Autodesk Inventor part; units mm, degrees
ref_plane "Work Plane1" through (-2.5, 0, -1.5) normal (0, 0, -1) x (-1, 0, 0)
ref_plane "Work Plane2" through (3.625, 2, -19.5) normal (0, 0, -1) x (-1, 0, 0)
ref_plane "YZ Plane" through (0, 0, 0) normal (1, 0, 0) x (0, 1, 0)
sketch "Sketch2" plane through (0, 0, 0) normal (0, 0, 1) x (1, 0, 0)
  circle A0 centre (2.5, 0) radius 1.5
  circle A1 centre (-2.5, 0) radius 1.5
  arc A2 (-1.9231, 1.3846) -> (1.9231, 1.3846) centre (0, 6) ccw
  arc A3 (1.9231, -1.3846) -> (-1.9231, -1.3846) centre (0, -6) ccw
  circle A4 centre (2.5, 0) radius 0.75
  circle A5 centre (-2.5, 0) radius 0.75
  point P0 (0, 0)
  dimension "d0" = 3
  dimension "d1" = 3
  dimension "d2" = 6
  dimension "d3" = 6
  dimension "d4" = 2.5
  dimension "d5" = 2.5
  dimension "d6" = 1.5
  dimension "d7" = 1.5
extrude "Extrusion2" add sketch "Sketch2" along normal blind 0.8
sketch "Sketch3" plane through (0, 0, 0) normal (0, 0, -1) x (-1, 0, 0)
  arc A0 (1.9231, -1.3846) -> (-1.9231, -1.3846) centre (0, -6) ccw
  arc A1 (1.9231, -1.3846) -> (1.9231, 1.3846) centre (2.5, 0) ccw
  arc A2 (-1.9231, 1.3846) -> (1.9231, 1.3846) centre (0, 6) ccw
  arc A3 (-1.9231, 1.3846) -> (-1.9231, -1.3846) centre (-2.5, 0) ccw
  circle A4 centre (-2.5, 0) radius 0.75
  circle A5 centre (2.5, 0) radius 0.75
  circle A6 centre (-2.5, 0) radius 1.125
  line L0 (-3.625, 2) -> (-1.375, 2)
  line L1 (-1.375, 2) -> (-1.375, 0)
  line L2 (-3.625, 0) -> (-3.625, 2)
  line L3 (0, -8.4) -> (0, 8.4)
  point P0 (0, 0)
  point P1 (-3.4922, 1.125)
  point P2 (-3.625, 0.9922)
  point P3 (-1.375, 1.1928)
  dimension "d12" = 2.25
  dimension "d16" = 1.5
  dimension "d20" = 2
extrude "Extrusion3" add sketch "Sketch3" along normal blind 1.5 contours L2 L0 L1 A2 A3 | A3 A2 L1 A6 L2 | A6
mirror "Mirror1" about plane through (0, 0, 0) normal (1, 0, 0) of "Extrusion3"
ref_plane "Work Plane1" through (-2.5, 0, -1.5) normal (0, 0, -1) x (-1, 0, 0)
mirror "Mirror2" about plane through (-2.5, 0, -1.5) normal (0, 0, -1) of "Extrusion3", "Mirror1", "Extrusion2"
sketch "Sketch4" plane through (1.375, 2, 0) normal (0, 1, 0) x (1, 0, 0)
  line L0 (-5, -4.5) -> (2.25, -4.5)
  line L1 (2.25, -4.5) -> (2.25, 1.5)
  line L2 (-5, 1.5) -> (-5, -4.5)
  line L3 (-2.75, 0) -> (-5, 0)
  line L4 (-2.75, 0) -> (-2.75, 3)
  line L5 (-2.75, 3) -> (-5, 3)
  line L6 (-5, 0) -> (-5, 3)
  line L7 (0, 0) -> (2.25, 0)
  line L8 (2.25, 0) -> (2.25, 3)
  line L9 (0, 3) -> (2.25, 3)
  line L10 (0, 0) -> (0, 3)
  line L11 (-5, 0) -> (-5, 3)
  line L12 (2.25, 0) -> (2.25, 3)
  line L13 (2.25, 1.5) -> (-5, 1.5)
  line L14 (2.25, 1.5) -> (-5, 1.5)
  line L15 (-5, 1.5) -> (-5, 19.5)
  line L16 (-5, 19.5) -> (2.25, 19.5)
  line L17 (2.25, 19.5) -> (2.25, 1.5)
  point P0 (-1.375, 0)
  point P1 (2.25, 1.5)
  point P2 (2.25, 3)
  dimension "d22" = 18
  dimension "d23" = 6
extrude "Extrusion4" add sketch "Sketch4" along normal blind 1.5
sketch "Sketch5" plane through (1.375, 3.5, 0) normal (0, 1, 0) x (1, 0, 0)
  line L0 (1.5, -1.5) -> (-4.25, -1.5)
  line L1 (-4.25, -1.5) -> (-4.25, -3.5)
  line L2 (-4.25, -3.5) -> (1.5, -3.5)
  line L3 (1.5, -3.5) -> (1.5, -1.5)
  line L4 (-5, -4.5) -> (2.25, -4.5)
  line L5 (2.25, -4.5) -> (2.25, 19.5)
  line L6 (2.25, 19.5) -> (-5, 19.5)
  line L7 (-5, 19.5) -> (-5, -4.5)
  point P0 (-1.375, 0)
  dimension "d26" = 5.75
  dimension "d27" = 7.25
  dimension "d28" = 2
  dimension "d29" = 0.75
  dimension "d30" = 1
extrude "Extrusion5" add sketch "Sketch5" along normal blind 1 contours L3 L2 L1 L0
pattern_linear "Rectangular Pattern1" count 5 spacing 4 along (0, 0, -1) of "Extrusion5"
ref_plane "Work Plane2" through (3.625, 2, -19.5) normal (0, 0, -1) x (-1, 0, 0)
mirror "Mirror3" about plane through (3.625, 2, -19.5) normal (0, 0, -1) of "Extrusion4", "Extrusion3", "Mirror1", "Extrusion2", "Mirror2", "Extrusion5", "Rectangular Pattern1"
equation "\"d1\" = d0"
equation "\"d7\" = d6"
equation "\"d12\" = d16 + 0.5 * d13"
equation "\"d29\" = -0.5 * d26 + 0.5 * d27"
properties part number "McCrea_CHAIN_INK_WALLE"
Here's how the part is built. I have some questions about the finished solid (model axes, mm). A direction names the side the tool comes from. Round coordinates to 2 decimals unless told otherwise and drop trailing zeros. Order: outer loops, then holes, each group sorted by start corner. A loop starts at its lowest first (then second) coordinate and runs counter-clockwise, first axis right, second up. Notation, with made-up numbers: (-25, 4.25) -> (-18, 4.25) arc R35 ccw to (-18, 40.25) -> close; hole circle Ø7 at (42, 61). An arc over 180 degrees is marked (long way). Use CSV: the item, a comma, the result in double quotes.
1. I need wall thicknesses on line 1 along Y through (x, z) = (2.5, -35.55); line 2 along Z through (x, y) = (0.25, -0.1); line 3 along Y through (x, z) = (-2.5, -36.7) (3 decimals). Which ranges of each line are inside material? Lowest first, please.
Recorded:
line 1,"y = -1.5 to -0.75, 0.75 to 1.5, 2 to 3.5"
line 2,"z = -39.8 to -39, -36 to -35.2, -3.8 to -3, 0 to 0.8"
line 3,"y = -1.125 to -0.75, 0.75 to 4.5"
2. I'm going to push flat-ended pins straight in: P1, Ø0.8, axis at y = 4, z = -2, coming from the -X side (3 decimals); P2, Ø0.8, axis at x = 1, y = 4, coming from the -Z side; P3, Ø0.8, axis at x = 1.5, y = 0, coming from the -Z side. Where does each tip first touch, or does it pass through?
Recorded:
P1,"stops at x = -2.875"
P2,"stops at z = -42.5"
P3,"stops at z = -39.8"
3. Thinking about a two-plate mould opening in Y: for faces 5 (the face through (0, 4.5, -2)), 6 (the face through (0, 0, -36)), 7 (the face through (-2.5, 1.7, -39)), which applies, pulls with the +Y half, pulls with the -Y half, needs draft (parallel to the pull), parting line crosses it, or undercut?
Recorded:
face 5,"pulls with the +Y half"
face 6,"needs draft"
face 7,"undercut"
4. Which directions (+Z, -Z, +X, -X, +Y, -Y) give clear straight access to the entire face, cutting with the end or side of a thin tool? Please do faces 1 (the face through (0, 0, 0.8)), 2 (the face through (2.875, 4, -1)), 3 (the face through (-4, 0, 0.4)), 4 (the face through (-2.875, 4, -2)).
Recorded:
face 1,"+Z, +X, -X, -Y"
face 2,"+Z, -Z, +X, +Y"
face 3,"+Z"
face 4,"+Z, -Z, -X, +Y"
5. I want a section at A-A on y = 4. Give the number of separate pieces and of enclosed holes in the cut face, and give its area (3 significant figures).
Recorded:
separate pieces,"10"
enclosed holes,"0"
area,"115 mm2"
6. I want a section at B-B on z = -22. List the corners of the cut face in (x, y) for me (3 decimals).
Recorded:
outline,"(-3.625, 2) -> (3.625, 2) -> (3.625, 3.5) -> (-3.625, 3.5) -> close"
